Read the model definition and answer for the solid it produces. Units are mm, in the model's axes. A direction names the side the tool comes from. Round coordinates to 2 decimals unless told otherwise and drop trailing zeros. Order: outer loops, then holes, each group sorted by start corner. A loop starts at its lowest first (then second) coordinate and runs counter-clockwise, first axis right, second up. Notation, with made-up numbers: (54, 65.25) - (106, 65.25) arc R33 ccw to (106, 99.25) - close; hole circle Ø6 at (33.5, -12). An arc over 180 degrees is marked (long way). Answer as a JSON object with one key per item and string values. Group by question number.
Q1. A cutting plane is placed at C-C on z = -22.5. Determine the outline of the cut face in (x, y).
Q2. A cutting plane is placed at D-D on x = -8. Determine the outline of the cut face in (y, z), and give its area (3 significant figures).
Q3. Given pin 1 Ø2 at (x, y) = (-91, -9.5) entering from -Z; pin 2 Ø2.5 at (x, y) = (-79.5, -98.5) entering from -Z, each flat-ended and moving along its own axis, determine where each tip first touches the part or whether it passes through.
Q4. Consider line 1 (Y direction, x = -56, z = 1); line 2 (X direction, y = -73.5, z = -24); line 3 (Y direction, x = -54, z = -7.5). Determine where each line is inside the solid, lowest interval first.
Q5. A cutting plane is placed at A-A on y = -33. Determine the outline of the cut face in (x, z), and give its area (3 significant figures).
Q6. A tool of negligible diameter and unlimited length cuts with its end or side. For faces 1 (the flat face through (-32, -59, -20)), 2 (the flat face through (-83, -100, -4)), 3 (the flat face through (-74, -99, -5)), from which of +Z, -Z, +X, -X, +Y, -Y can it reach the whole face along a straight path? Write none if from no direction.
Q7. A cutting plane is placed at B-B on x = -56. Determine the outline of the cut face in (y, z), and give its area (3 significant figures).
```python
from build123d import *

# Parameters (mm, degrees)
SKETCH018_W           = 32
SKETCH018_H           = 32
EXTRUDE017_DEPTH      = 10
SKETCH_R              = 2.1
EXTRUDE002_DEPTH      = 20
SKETCH003_R           = 4.5
EXTRUDE003_DEPTH      = 3
EXTRUDE003_DEPTH_BACK = 1
EXTRUDE001_DEPTH      = 2
SKETCH011_R           = 1.1
EXTRUDE010_DEPTH      = 25
EXTRUDE_DEPTH         = 30


with BuildPart() as cone001:
    # Cone001 → Cone001 (revolve)
    with BuildSketch(Plane(origin=(-91.1, -9.1, -19.4), x_dir=(1, 0, 0), z_dir=(0, -1, 0))):
        Polygon((0, 0), (2.1, 0), (6, 20), (0, 20), align=None)
    revolve(axis=Axis((-91.1, -9.1, -19.4), (0, 0, 1)))


with BuildPart() as cone002:
    # Cone002 → Cone002 (revolve)
    with BuildSketch(Plane(origin=(-33, -58.1, -19.4), x_dir=(1, 0, 0), z_dir=(0, -1, 0))):
        Polygon((0, 0), (2.1, 0), (6, 20), (0, 20), align=None)
    revolve(axis=Axis((-33, -58.1, -19.4), (0, 0, 1)))


with BuildPart() as cone003:
    # Cone003 → Cone003 (revolve)
    with BuildSketch(Plane(origin=(-90.9, -58.2, -19.4), x_dir=(1, 0, 0), z_dir=(0, -1, 0))):
        Polygon((0, 0), (2.1, 0), (6, 20), (0, 20), align=None)
    revolve(axis=Axis((-90.9, -58.2, -19.4), (0, 0, 1)))


with BuildPart() as extrude017:
    # Sketch018 (on Face8 of Fusion) → Extrude017 (new body, symmetric)
    with BuildSketch(Plane.XZ.offset(100)):
        with Locations((-74, -21)):
            Rectangle(SKETCH018_W, SKETCH018_H)
    extrude(amount=EXTRUDE017_DEPTH, both=True)


with BuildPart() as extrude002:
    # Sketch → Extrude002 (new body)
    with BuildSketch(Plane.XY):
        with Locations((-91, -9)):
            Circle(SKETCH_R)
        with Locations((-33, -9)):
            Circle(SKETCH_R)
        with Locations((-33, -58)):
            Circle(SKETCH_R)
        with Locations((-91, -58)):
            Circle(SKETCH_R)
    extrude(amount=-EXTRUDE002_DEPTH)


with BuildPart() as extrude003:
    # Sketch003 → Extrude003 (new body, two sides)
    with BuildSketch(Plane.XY) as extrude003_sk:
        with Locations((-78, -19)):
            Circle(SKETCH003_R)
        with Locations((-67, -19)):
            Circle(SKETCH003_R)
        with Locations((-56, -19)):
            Circle(SKETCH003_R)
        with Locations((-45, -19)):
            Circle(SKETCH003_R)
        with Locations((-78, -33)):
            Circle(SKETCH003_R)
        with Locations((-67, -33)):
            Circle(SKETCH003_R)
        with Locations((-56, -33)):
            Circle(SKETCH003_R)
        with Locations((-45, -33)):
            Circle(SKETCH003_R)
        with Locations((-78, -47)):
            Circle(SKETCH003_R)
        with Locations((-67, -47)):
            Circle(SKETCH003_R)
        with Locations((-56, -47)):
            Circle(SKETCH003_R)
        with Locations((-45, -47)):
            Circle(SKETCH003_R)
    extrude(amount=EXTRUDE003_DEPTH)
    extrude(extrude003_sk.sketch, amount=-EXTRUDE003_DEPTH_BACK)


with BuildPart() as cut:
    # Sketch002 → Extrude001 (new body)
    with BuildSketch(Plane.XY):
        Polygon((0, 0), (0, -86), (-50, -100), (-104, -100), (-104, 0), align=None)
    extrude(amount=EXTRUDE001_DEPTH)

    # Cut: cut Extrude003
    add(extrude003.part, mode=Mode.SUBTRACT)


with BuildPart() as extrude010:
    # Sketch011 → Extrude010 (new body)
    with BuildSketch(Plane.XY):
        with Locations((-91, -9)):
            Circle(SKETCH011_R)
        with Locations((-33, -9)):
            Circle(SKETCH011_R)
        with Locations((-33, -58)):
            Circle(SKETCH011_R)
        with Locations((-91, -58)):
            Circle(SKETCH011_R)
    extrude(amount=-EXTRUDE010_DEPTH)


with BuildPart() as cut004:
    # Sketch001 → Extrude (new body)
    with BuildSketch(Plane.XY):
        Polygon((0, 0), (0, -86), (-50, -100), (-104, -100), (-104, 0), align=None)
        Polygon((-3, -3), (-3, -83.84), (-50, -97), (-101, -97), (-101, -3), align=None, mode=Mode.SUBTRACT)
    extrude(amount=-EXTRUDE_DEPTH)

    # Fusion: union Extrude002, Cut, Extrude010
    add(extrude002.part)
    add(cut.part)
    add(extrude010.part)

    # Cut004: cut Extrude017
    add(extrude017.part, mode=Mode.SUBTRACT)


with BuildPart() as fusion003:
    # Cone → Cone (revolve)
    with BuildSketch(Plane(origin=(-33, -9.1, -19.4), x_dir=(1, 0, 0), z_dir=(0, -1, 0))):
        Polygon((0, 0), (2.1, 0), (6, 20), (0, 20), align=None)
    revolve(axis=Axis((-33, -9.1, -19.4), (0, 0, 1)))

    # Fusion003: union Cone001, Cone002, Cone003, Cut004
    add(cone001.part)
    add(cone002.part)
    add(cone003.part)
    add(cut004.part)


solid = fusion003.part
```
Result set:
{
 "1": {"outline": "(-104, -100) - (-90, -100) - (-90, -97) - (-101, -97) - (-101, -3) - (-3, -3) - (-3, -83.84) - (-50, -97) - (-58, -97) - (-58, -100) - (-50, -100) - (0, -86) - (0, 0) - (-104, 0) - close; circle Ø2.2 at (-91, -58); circle Ø2.2 at (-91, -9); circle Ø2.2 at (-33, -58); circle Ø2.2 at (-33, -9)"},
 "2": {"outline": "(-88.24, -30) - (-85.24, -30) - (-85.24, 0) - (-3, 0) - (-3, -30) - (0, -30) - (0, 2) - (-88.24, 2) - close", "area": "356 mm²"},
 "3": {"pin 1": "stops at z = -25", "pin 2": "stops at z = -5"},
 "4": {"line 1": "y = -100 to -51.5, -42.5 to -37.5, -28.5 to -23.5, -14.5 to 0", "line 2": "x = -104 to -101, -3 to 0", "line 3": "y = -100 to -97, -3 to 0"},
 "5": {"outline": "(-104, -30) - (-101, -30) - (-101, 0) - (-82.5, 0) - (-82.5, 2) - (-104, 2) - close; (-73.5, 0) - (-71.5, 0) - (-71.5, 2) - (-73.5, 2) - close; (-62.5, 0) - (-60.5, 0) - (-60.5, 2) - (-62.5, 2) - close; (-51.5, 0) - (-49.5, 0) - (-49.5, 2) - (-51.5, 2) - close; (-40.5, 0) - (-3, 0) - (-3, -30) - (0, -30) - (0, 2) - (-40.5, 2) - close", "area": "316 mm²"},
 "6": {"face 1": "-Z", "face 2": "+Z, -Z, +X, -X, -Y", "face 3": "-Z, -Y"},
 "7": {"outline": "(-100, -30) - (-97, -30) - (-97, 0) - (-51.5, 0) - (-51.5, 2) - (-100, 2) - close; (-42.5, 0) - (-37.5, 0) - (-37.5, 2) - (-42.5, 2) - close; (-28.5, 0) - (-23.5, 0) - (-23.5, 2) - (-28.5, 2) - close; (-14.5, 0) - (-3, 0) - (-3, -30) - (0, -30) - (0, 2) - (-14.5, 2) - close", "area": "326 mm²"}
}
